The model under review builds one solid part; all positions refer to its coordinate system, in mm. Face numbers are marked on the shaded views. A direction names the side the tool comes from. Round coordinates to 2 decimals unless told otherwise and drop trailing zeros. Write each loop counter-clockwise with the first axis right and the second up, starting at its lowest first coordinate (ties: lowest second). Pieces come first, ordered by that corner, then holes. Notation, with made-up numbers: M -4.75,65 L 29.25,65 A23 cw 29.25,97 Z; hole C 43.5,36 d1. An arc over 180 degrees is marked long. One line per item, written item: value. Start each with the question number.
1) For P1, Ø4, axis at x = -11.5, z = -53, coming from the +Y side; P2, Ø6, axis at y = 4, z = -116.5, coming from the +X side; P3, Ø10, axis at x = 9, z = -87, coming from the +Y side, all flat-tipped, find the tip position at first contact; note any pin that passes through.
2) Tool access review of the marked faces 4 and 5: name each direction out of +Z, -Z, +X, -X, +Y, -Y from which nothing blocks a thin tool from reaching the whole face with its end or side.
3) Mouldability with a two-part tool opening along X and no side actions: class the marked faces 1, 2 and 3 as +X half, -X half, draft (parallel to the pull), parting line (faces both ways), or undercut.
4) Take a section at A-A, the plane z = -120.5. Write out the cut boundary in (x, y).
5) Take a section at D-D, the plane z = -102.5. Write out the cut boundary in (x, y), and give its area (3 significant figures).
6) Wall thickness on probe 1 along Z at (x, y) = (3.75, 1.5); probe 2 along Z at (x, y) = (9.5, -0.75); probe 3 along Z at (x, y) = (9.75, -6.25): over which ranges is each line inside the solid? List them lowest first.
7) Take a section at C-C, the plane z = -32. Write out the cut boundary in (x, y), and give its area (3 significant figures).
8) Take a section at B-B, the plane y = 9.25. Write out the cut boundary in (x, z).
from build123d import *

# Parameters (mm, degrees)
BOSS_EXTRUDE3_DEPTH = 20
SKETCH4_W           = 12
SKETCH4_H           = 7.1
CUT_EXTRUDE1_DEPTH  = 132.719398723


with BuildPart() as part:
    # Sketch2 → Revolve4 (revolve)
    with BuildSketch(Plane(origin=(0, 0, 0), x_dir=(1, 0, 0), z_dir=(0, 1, 0))):
        Polygon((0, 0), (8, 0), (8, 50), (10.5, 50), (10.5, 100), (15, 100), (15, 110), (0, 110), align=None)
    revolve(axis=Axis((0, 0, 0), (0, 0, -1)))

    # Sketch3 → Boss-Extrude3 (add)
    with BuildSketch(Plane(origin=(0, 0, -110), x_dir=(-1, 0, 0), z_dir=(0, 0, -1))):
        with BuildLine():
            Line((-14, 0), (-12, 0))
            ThreePointArc((-12, 0), (-11.983554417, 0.628031475), (-11.934262744, 1.254341559))
            Line((-11.934262744, 1.254341559), (-13.923306535, 1.463398486))
            ThreePointArc((-13.923306535, 1.463398486), (-13.980813487, 0.732703387), (-14, 0))
        make_face()
        with BuildLine():
            Line((14, 0), (12, 0))
            ThreePointArc((12, 0), (0, -12), (-12, 0))
            Line((-12, 0), (-14, 0))
            ThreePointArc((-14, 0), (0, -14), (14, 0))
        make_face()
        with BuildLine():
            ThreePointArc((11.934262744, 1.254341559), (11.983554417, 0.628031475), (12, 0))
            Line((12, 0), (14, 0))
            ThreePointArc((14, 0), (13.980813487, 0.732703387), (13.923306535, 1.463398486))
            Line((13.923306535, 1.463398486), (11.934262744, 1.254341559))
        make_face()
    extrude(amount=BOSS_EXTRUDE3_DEPTH)

    # Sketch4 → Cut-Extrude1 (cut, through all)
    with BuildSketch(Plane(origin=(0, 0, 0), x_dir=(0, 0, -1), z_dir=(1, 0, 0))):
        with Locations((72, 0)):
            Rectangle(SKETCH4_W, SKETCH4_H)
    extrude(amount=CUT_EXTRUDE1_DEPTH, mode=Mode.SUBTRACT)


solid = part.part
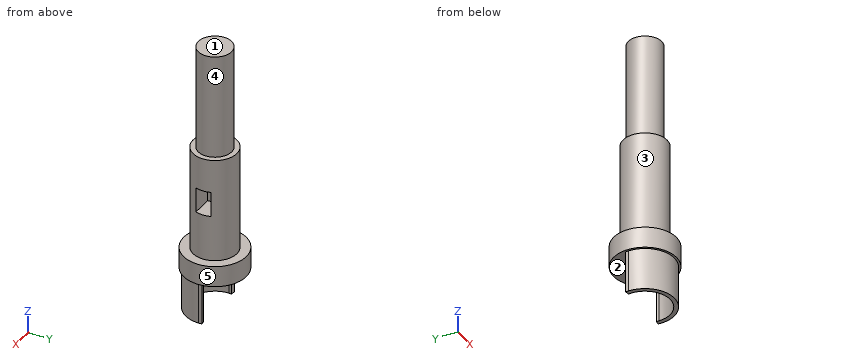
Checked values:
1. P1: stops at y = 4.47
1. P2: stops at x = 13.96
1. P3: stops at y = 9.71
2. face 4: +Z
2. face 5: +Z, -Z
3. face 1: draft
3. face 2: undercut
3. face 3: parting line
4. outline: M -13.92,1.46 A14 ccw long 13.92,1.46 L 11.93,1.25 A12 cw long -11.93,1.25 Z
5. outline: C 0,0 d30
5. area: 707 mm2
6. probe 1: z = -110 to -78, -66 to 0
6. probe 2: z = -110 to -78, -66 to -50
6. probe 3: z = -110 to -100
7. outline: C 0,0 d16
7. area: 201 mm2
8. outline: M -11.81,-110 L 11.81,-110 L 11.81,-100 L 4.97,-100 L 4.97,-50 L -4.97,-50 L -4.97,-100 L -11.81,-100 Z
